from build123d import *

# Parameters (mm, degrees)
F0_W     = 1066.8
F0_H     = 685.8
F1_DEPTH = 19.05
F2_W     = 19.05
F2_H     = 666.75
F2_H_2   = 664.6272460461
F3_DEPTH = 406.4
F5_W     = 1066.8
F5_H     = 685.8
F6_DEPTH = 19.05


with BuildPart() as f1:
    # F0 (on Top) → F1 (new body)
    with BuildSketch(Plane.XY):
        Rectangle(F0_W, F0_H)
    extrude(amount=F1_DEPTH)

    # F2 (on face) → F3 (join)
    with BuildSketch(Plane.XY.offset(19.05)):
        with Locations((-523.875, -9.525)):
            Rectangle(F2_W, F2_H)
        Polygon((-533.4, 323.85), (-514.35, 323.85), (514.35, 323.85), (533.4, 323.85), (533.4, 342.9), (-533.4, 342.9), align=None)
        with Locations((523.875, -9.525)):
            Rectangle(F2_W, F2_H)
        with Locations((-98.425, -10.586376977)):
            Rectangle(F2_W, F2_H_2)
    extrude(amount=F3_DEPTH)

    # F5 (on offset) → F6 (join)
    with BuildSketch(Plane.XY.offset(425.45)):
        Rectangle(F5_W, F5_H)
    extrude(amount=F6_DEPTH)


solid = f1.part
CAD build for the part. Positions are in the model's coordinates, mm. A direction names the side the tool comes from. Round coordinates to 2 decimals unless told otherwise and drop trailing zeros. Loops run counter-clockwise (first coordinate to the right, second up) from the corner with the lowest first, then second, coordinate; pieces in that order, holes last.
(1) Which spindle directions (+Z, -Z, +X, -X, +Y, -Y) get a long thin tool onto all of the face, cutting with end or side? Do faces 5 (the flat face through (-533.4, -5, 219)), 6 (the flat face through (-514.35, -14, 219)). Say none if no direction does.
(2) Cut at B-B (y = -279.5). Give the cut face in (x, z).
(3) Wall check: line 1 along X through (y, z) = (-95, 238); line 2 along Y through (x, z) = (-89, 97); line 3 along Z through (x, y) = (-6, 69). Give the ranges that are in metal, low to high.
(4) Two-plate mould, pull along Z, no slides. Class faces 1 (the flat face through (-107.95, -15, 219)), 2 (the flat face through (-161, -342.9, 7)), 3 (the flat face through (-7, 5, 0)), 4 (the flat face through (-7, 323.85, 219)): +Z half, -Z half, draft (parallel to the pull), parting line (faces both ways), or undercut.
(5) Cut at C-C (x = 394.5). Give the cut face in (y, z).
(6) Drop a flat-ended pin along its axis: pin 1 (4 mm diameter, centred on x = -368.5, z = 63, fed in from -Y). Give the stop position or say it passes through.
(7) Cut at A-A (z = 178). Give the cut face in (x, y), plus the area to 3 significant figures.
Findings below:
1. face 5: +Z, -Z, -X, +Y, -Y
1. face 6: -Y
2. outline: (-533.4, 0) - (533.4, 0) - (533.4, 444.5) - (-533.4, 444.5) - close; hole (-514.35, 19.05) - (-107.95, 19.05) - (-107.95, 425.45) - (-514.35, 425.45) - close; hole (-88.9, 19.05) - (514.35, 19.05) - (514.35, 425.45) - (-88.9, 425.45) - close
3. line 1: x = -533.4 to -514.35, -107.95 to -88.9, 514.35 to 533.4
3. line 2: y = -342.9 to 321.73, 323.85 to 342.9
3. line 3: z = 0 to 19.05, 425.45 to 444.5
4. face 1: undercut
4. face 2: draft
4. face 3: -Z half
4. face 4: undercut
5. outline: (-342.9, 0) - (342.9, 0) - (342.9, 444.5) - (-342.9, 444.5) - (-342.9, 425.45) - (323.85, 425.45) - (323.85, 19.05) - (-342.9, 19.05) - close
6. pin 1: stops at y = 323.85
7. outline: (-533.4, -342.9) - (-514.35, -342.9) - (-514.35, 323.85) - (514.35, 323.85) - (514.35, -342.9) - (533.4, -342.9) - (533.4, 342.9) - (-533.4, 342.9) - close; (-107.95, -342.9) - (-88.9, -342.9) - (-88.9, 321.73) - (-107.95, 321.73) - close
7. area: 58,400 mm2
